Could you check a few things on this drawing? It's one solid part, dimensions in mm from its lowest x, y, z. A direction names the side the tool comes from. Give positions to 0.01 mm unless a question says otherwise; leave off trailing zeros. Order: outer loops, then holes, each group sorted by start corner. A loop starts at its lowest first (then second) coordinate and runs counter-clockwise, first axis right, second up. Notation, with made-up numbers: M 89.25,-23.75 L 142.25,-23.75 A31 ccw 142.25,10.25 Z; hole C 34.5,-8.75 d2. An arc over 180 degrees is marked long. One line per item, written item: value. Start each with the question number.
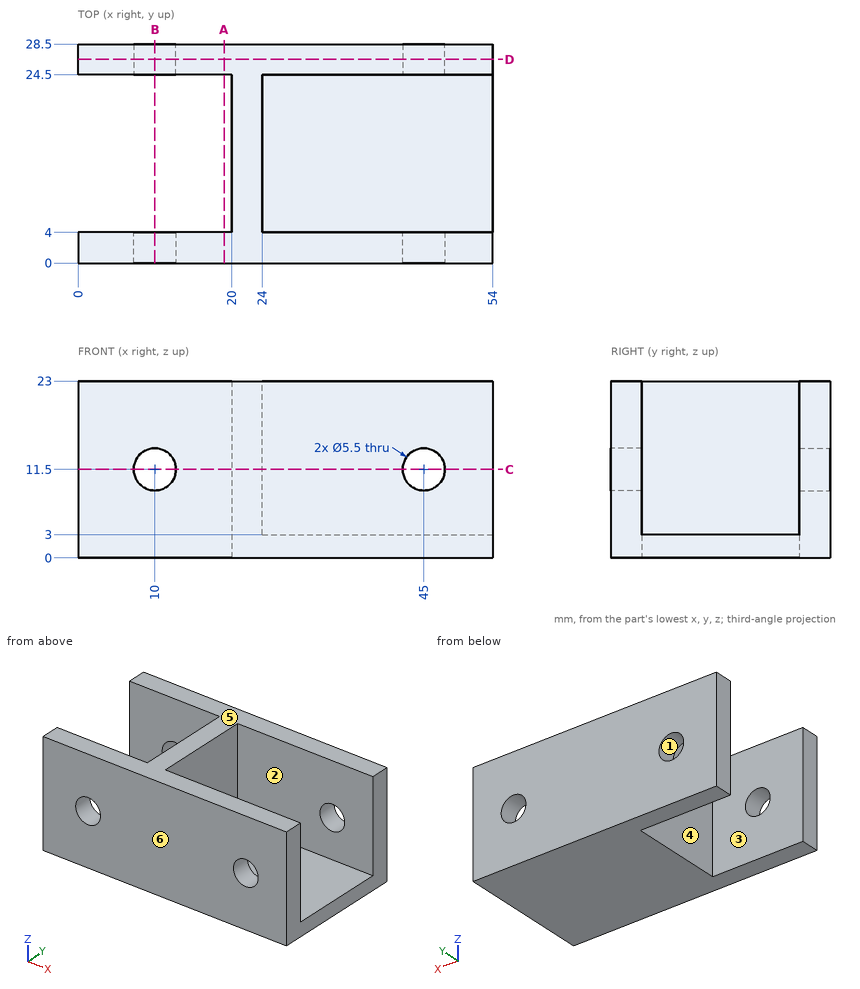
Item 1: I want a section at D-D on y = 26.5. Write out the boundary of the cut face in (x, z).
Item 2: I want a section at C-C on z = 11.5. Write out the boundary of the cut face in (x, y), plus the area to 3 significant figures.
Item 3: I want a section at A-A on x = 19. Write out the boundary of the cut face in (y, z), plus the area to 3 significant figures.
Item 4: We'd pull the mould along Y, two halves only. Please class the marked faces 4, 5 and 6: +Y half, -Y half, draft (parallel to the pull), parting line (faces both ways), or undercut.
Item 5: I want a section at B-B on x = 10. Write out the boundary of the cut face in (y, z), plus the area to 3 significant figures.
Item 6: For the marked faces 1, 2 and 3, which set-ups out of +Z, -Z, +X, -X, +Y, -Y let a thin tool reach every point of the face, with its end or its side?
Item 7: Please list where these lines run through material, in increasing order: probe 1 along X at (y, z) = (1.35, 11.5); probe 2 along Y at (x, z) = (36.5, 4.25); probe 3 along Z at (x, y) = (10, 25.4). Write a range as [from, to].
Item 8: Will these pins go through, and if not, where does the flat tip stop? P1, Ø10, axis at x = 45, z = 10, coming from the +Y side; P2, Ø5, axis at y = 8, z = 7.5, coming from the -X side; P3, Ø10, axis at x = 8, y = 19, coming from the -Z side.
Answer below:
1. outline: M 0,0 L 54,0 L 54,23 L 0,23 Z; hole C 10,11.5 d5.5; hole C 45,11.5 d5.5
2. outline: M 0,0 L 7.25,0 L 7.25,4 L 0,4 Z; M 0,24.5 L 7.25,24.5 L 7.25,28.5 L 0,28.5 Z; M 12.75,0 L 42.25,0 L 42.25,4 L 24,4 L 24,24.5 L 42.25,24.5 L 42.25,28.5 L 12.75,28.5 L 12.75,24.5 L 20,24.5 L 20,4 L 12.75,4 Z; M 47.75,0 L 54,0 L 54,4 L 47.75,4 Z; M 47.75,24.5 L 54,24.5 L 54,28.5 L 47.75,28.5 Z
2. area: 426 mm²
3. outline: M 0,0 L 4,0 L 4,23 L 0,23 Z; M 24.5,0 L 28.5,0 L 28.5,23 L 24.5,23 Z
3. area: 184 mm²
4. face 4: undercut
4. face 5: draft
4. face 6: -Y half
5. outline: M 0,0 L 4,0 L 4,8.75 L 0,8.75 Z; M 0,14.25 L 4,14.25 L 4,23 L 0,23 Z; M 24.5,0 L 28.5,0 L 28.5,8.75 L 24.5,8.75 Z; M 24.5,14.25 L 28.5,14.25 L 28.5,23 L 24.5,23 Z
5. area: 140 mm²
6. face 1: +Y, -Y
6. face 2: +Z, +X
6. face 3: +Z, -Z, -X
7. probe 1: x = [0, 7.25], [12.75, 42.25], [47.75, 54]
7. probe 2: y = [0, 4], [24.5, 28.5]
7. probe 3: z = [0, 8.75], [14.25, 23]
8. P1: stops at y = 28.5
8. P2: stops at x = 20
8. P3: passes through
